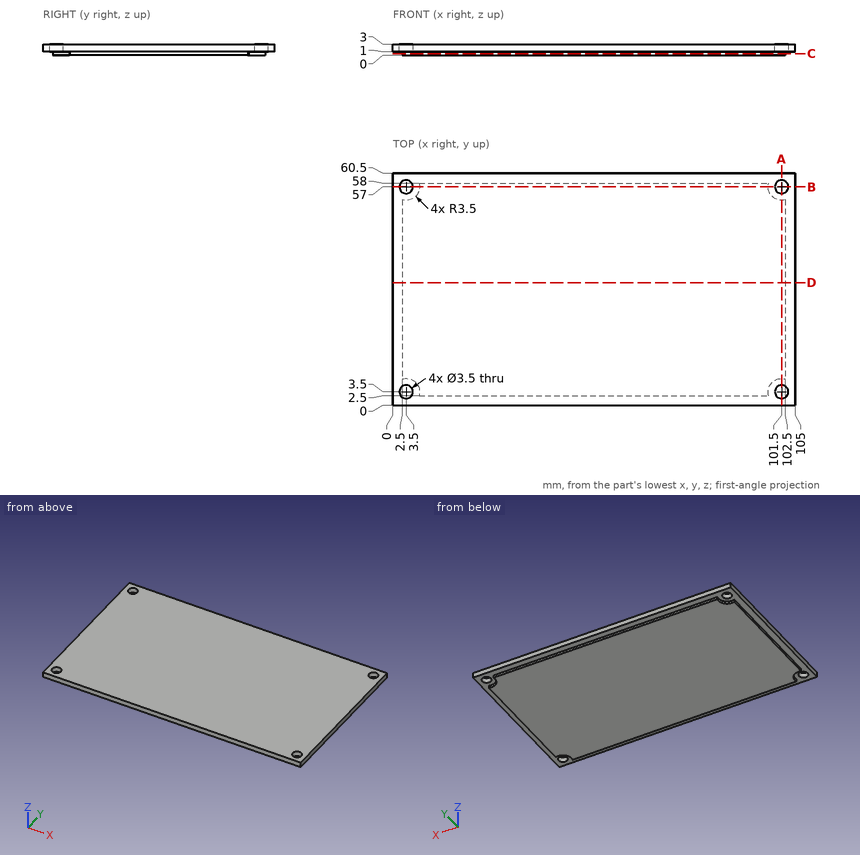
Check sheet for the drawn part. Datum: minimum x, y, z corner. Units: mm. Round coordinates to 2 decimals unless told otherwise and drop trailing zeros. Write each loop counter-clockwise with the first axis right and the second up, starting at its lowest first coordinate (ties: lowest second). Pieces come first, ordered by that corner, then holes. Notation, with made-up numbers: (-12, -7) - (27, -7) arc R21 cw to (27, 16) - close; hole circle Ø1 at (19, 69). An arc over 180 degrees is marked (long way). Write each question's results on one line, items separated by ' | '.
(1) Sectioned sample at A-A, the plane x = 101.5. Enter the section's corners in (y, z).
Computed:
outline: (0, 1) - (1.75, 1) - (1.75, 3) - (0, 3) - close; (5.25, 1) - (7, 1) - (7, 0) - (53.5, 0) - (53.5, 1) - (55.25, 1) - (55.25, 3) - (5.25, 3) - close; (58.75, 1) - (60.5, 1) - (60.5, 3) - (58.75, 3) - close
(2) Sectioned sample at B-B, the plane y = 57. Enter the section's corners in (x, z), plus the area to 3 significant figures.
Computed:
outline: (0, 1) - (1.75, 1) - (1.75, 3) - (0, 3) - close; (5.25, 1) - (7, 1) - (7, 0) - (98, 0) - (98, 1) - (99.75, 1) - (99.75, 3) - (5.25, 3) - close; (103.25, 1) - (105, 1) - (105, 3) - (103.25, 3) - close | area: 287 mm^2
(3) Sectioned sample at C-C, the plane z = 0.5. Enter the section's corners in (x, y).
Computed:
outline: (2.5, 6.85) arc R3.5 cw to (6.85, 2.5) - (98.15, 2.5) arc R3.5 cw to (102.5, 6.85) - (102.5, 53.65) arc R3.5 cw to (98.15, 58) - (6.85, 58) arc R3.5 cw to (2.5, 53.65) - close
(4) Sectioned sample at D-D, the plane y = 32. Enter the section's corners in (x, z), plus the area to 3 significant figures.
Computed:
outline: (0, 1) - (2.5, 1) - (2.5, 0) - (102.5, 0) - (102.5, 1) - (105, 1) - (105, 3) - (0, 3) - close | area: 310 mm^2
(5) Depth check by flat-ended pin: pin 1 Ø5.5 at (x, y) = (101.5, 3.5) entering from -Z; pin 2 Ø0.8 at (x, z) = (47.5, 0.5) entering from +Y; pin 3 Ø0.5 at (x, z) = (52.5, 0.5) entering from -Y. Enter the tip coordinate at first touch or a pass-through.
Computed:
pin 1: stops at z = 1 | pin 2: stops at y = 58 | pin 3: stops at y = 2.5
(6) Thickness scan on probe 1 along Y at (x, z) = (101.5, 1.95); probe 2 along X at (y, z) = (58, 1.5); probe 3 along Y at (x, z) = (75, 0.65). Record the ranges inside material, lowest first. Write a range as from..to.
Computed:
probe 1: y = 0..1.75, 5.25..55.25, 58.75..60.5 | probe 2: x = 0..2.06, 4.94..100.06, 102.94..105 | probe 3: y = 2.5..58
